```python
from build123d import *

# Parameters (mm, degrees)
F1_DEPTH = 7
F2_R     = 7.5
F3_DEPTH = 4
F4_R     = 1.975
F5_DEPTH = 16
F6_R     = 1.25
F7_DEPTH = 6


with BuildPart() as f1:
    # F0 (on Top) → F1 (new body)
    with BuildSketch(Plane.XY):
        with BuildLine():
            ThreePointArc((2.418677, -1.6), (2.9, 0), (2.418677, 1.6))
            Line((2.418677, 1.6), (-2.418677, 1.6))
            ThreePointArc((-2.418677, 1.6), (-2.9, 0), (-2.418677, -1.6))
            Line((-2.418677, -1.6), (2.418677, -1.6))
        make_face()
    extrude(amount=F1_DEPTH)

    # F2 (on face) → F3 (join)
    with BuildSketch(Plane(origin=(0, 0, 0), x_dir=(1, 0, 0), z_dir=(0, 0, -1))):
        Circle(F2_R)
    extrude(amount=F3_DEPTH)

    # F4 (on face) → F5 (join)
    with BuildSketch(Plane(origin=(0, 0, -4), x_dir=(1, 0, 0), z_dir=(0, 0, -1))):
        Circle(F4_R)
    extrude(amount=F5_DEPTH)

    # F6 (on face) → F7 (cut)
    with BuildSketch(Plane(origin=(0, 0, -20), x_dir=(1, 0, 0), z_dir=(0, 0, -1))):
        Circle(F6_R)
    extrude(amount=-F7_DEPTH, mode=Mode.SUBTRACT)


solid = f1.part
```
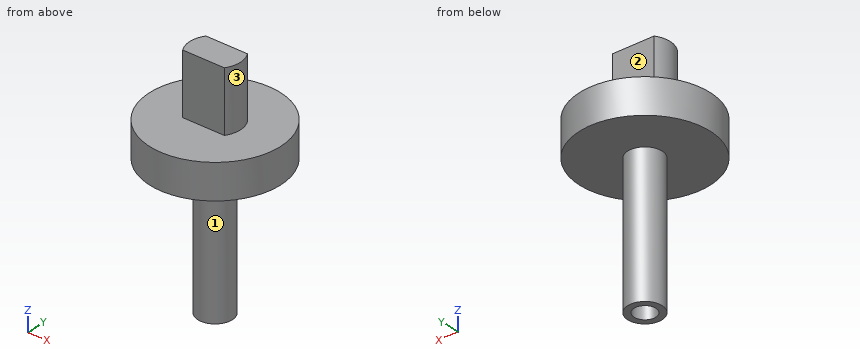
Verification items for the finished model (mm, model axes). Face numbers are marked on the shaded views. A direction names the side the tool comes from. Coordinates: 2 decimals unless noted, no trailing zeros. Loops run counter-clockwise (first coordinate to the right, second up) from the corner with the lowest first, then second, coordinate; pieces in that order, holes last. Notation, with made-up numbers: (-17.5, 3) -> (-5.5, 3) arc R15 cw to (-5.5, 19) -> close; hole circle Ø5 at (4, -24). An arc over 180 degrees is marked (long way). Put each result on its own line as item: value.
1. Tool access check on the marked faces 1, 2 and 3. Record the directions out of +Z, -Z, +X, -X, +Y, -Y that give a thin tool (end or side, any length) a straight path to the whole face; none if there is none.
Result set:
face 1: -Z
face 2: +Z, +X, -X, +Y
face 3: +Z, +X
2. Section check B-B, the plane x = 0. Record the boundary of the cut face in (y, z) (3 decimals).
Result set:
outline: (-7.5, -4) -> (-1.975, -4) -> (-1.975, -20) -> (-1.25, -20) -> (-1.25, -14) -> (1.25, -14) -> (1.25, -20) -> (1.975, -20) -> (1.975, -4) -> (7.5, -4) -> (7.5, 0) -> (1.6, 0) -> (1.6, 7) -> (-1.6, 7) -> (-1.6, 0) -> (-7.5, 0) -> close
3. Section check C-C, the plane z = -15.75. Record the boundary of the cut face in (x, y) (3 decimals), then the cut area to 3 significant figures.
Result set:
outline: circle Ø3.95 at (0, 0); hole circle Ø2.5 at (0, 0)
area: 7.35 mm^2
4. Section check D-D, the plane z = 2.5. Record the boundary of the cut face in (x, y), then the cut area to 3 significant figures.
Result set:
outline: (-2.42, -1.6) -> (2.42, -1.6) arc R2.9 ccw to (2.42, 1.6) -> (-2.42, 1.6) arc R2.9 ccw to start
area: 17.6 mm^2
5. Gauge pin test, flat ends, axial feed: P1, Ø3, axis at x = 3.5, y = -2, coming from the +Z side; P2, Ø2.5, axis at x = 1, z = 2.5, coming from the +Y side; P3, Ø4, axis at y = -1.5, z = -15, coming from the -X side (3 decimals); P4, Ø4, axis at x = -4.5, y = -4, coming from the -Z side. Record the tip position at first contact, or that the pin passes through.
Result set:
P1: stops at z = 7
P2: stops at y = 1.6
P3: stops at x = -1.975
P4: stops at z = -4
6. Section check A-A, the plane y = 0. Record the boundary of the cut face in (x, z) (3 decimals).
Result set:
outline: (-7.5, -4) -> (-1.975, -4) -> (-1.975, -20) -> (-1.25, -20) -> (-1.25, -14) -> (1.25, -14) -> (1.25, -20) -> (1.975, -20) -> (1.975, -4) -> (7.5, -4) -> (7.5, 0) -> (2.9, 0) -> (2.9, 7) -> (-2.9, 7) -> (-2.9, 0) -> (-7.5, 0) -> close
7. Thickness scan on line 1 (Y direction, x = 0, z = -15.85) (3 decimals); line 2 (Z direction, x = 1, y = 2.5). Record the ranges inside material, lowest first.
Result set:
line 1: y = -1.975 to -1.25, 1.25 to 1.975
line 2: z = -4 to 0
